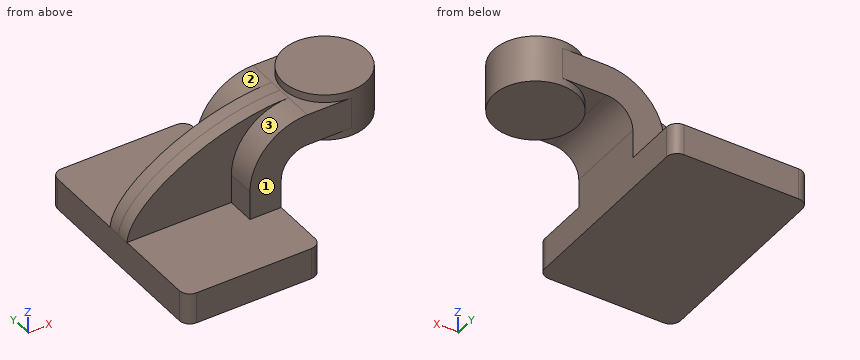
```python
from build123d import *

# Parameters (mm, degrees)
F1_DEPTH = 63.5
F0_W     = 25.4
F0_H     = 19.05
F2_DEPTH = 25.4
F3_DEPTH = 7.9375
F5_R     = 6.35


with BuildPart() as f1:
    # F0 (on Front) → F1 (new body, symmetric)
    with BuildSketch(Plane.XZ):
        Polygon((-41.275, -9.525), (41.275, -9.525), (41.275, 9.525), (22.225, 9.525), (-41.275, 9.525), align=None)
    extrude(amount=F1_DEPTH, both=True)

    # F0 (on Front) → F2 (join, symmetric)
    with BuildSketch(Plane.XZ):
        with BuildLine():
            Line((22.225, 9.525), (41.275, 9.525))
            Line((41.275, 9.525), (41.275, 27.0002))
            ThreePointArc((41.275, 27.0002), (45.9246798487, 38.2255201513), (57.15, 42.8752))
            Line((57.15, 42.8752), (58.7173181552, 42.8752))
            Line((58.7173181552, 42.8752), (58.7173181552, 61.9252))
            Line((58.7173181552, 61.9252), (57.15, 61.9252))
            ThreePointArc((57.15, 61.9252), (32.4542956671, 51.6959043329), (22.225, 27.0002))
            Line((22.225, 27.0002), (22.225, 9.525))
        make_face()
        with Locations((71.4173181552, 52.4002)):
            Rectangle(F0_W, F0_H)
    extrude(amount=F2_DEPTH, both=True)

    # F0 (on Front) → F3 (join, symmetric)
    with BuildSketch(Plane.XZ):
        with BuildLine():
            add(Edge.make_bspline(
                [(-41.275, 9.525), (-39.4876301289, 34.0806692839), (13.6961471289, 62.1632300317), (57.15, 61.9252)],
                knots=[0, 0, 0, 0, 111.5045361635, 111.5045361635, 111.5045361635, 111.5045361635], degree=3))
            Line((-41.275, 9.525), (22.225, 9.525))
            Line((22.225, 9.525), (22.225, 27.0002))
            ThreePointArc((22.225, 27.0002), (32.4542956671, 51.6959043329), (57.15, 61.9252))
        make_face()
    extrude(amount=F3_DEPTH, both=True)

    # F0 (on Front) → F4 (revolve)
    with BuildSketch(Plane.XZ):
        Polygon((84.1173181552, 66.675), (84.1173181552, 61.9252), (84.1173181552, 42.8752), (84.1173181552, 38.1), (109.5173181552, 38.1), (109.5173181552, 66.675), align=None)
    revolve(axis=Axis((84.1173181552, 0, 52.3875), (0, 0, 1)))

    # F5
    f5_edges = [f1.edges().sort_by_distance(p)[0] for p in [
        (41.275, -63.5, 0),
        (-41.275, -63.5, 0),
        (41.275, 63.5, 0),
        (-41.275, 63.5, 0),
    ]]
    fillet(f5_edges, radius=F5_R)


solid = f1.part
```
CAD build for the part. Positions are in the model's coordinates, mm. Face numbers are marked on the shaded views. A direction names the side the tool comes from. Round coordinates to 2 decimals unless told otherwise and drop trailing zeros. Write each loop counter-clockwise with the first axis right and the second up, starting at its lowest first coordinate (ties: lowest second). Pieces come first, ordered by that corner, then holes. Notation, with made-up numbers: (59, 80.25) - (90, 80.25) arc R27 cw to (90, 117.25) - close; hole circle Ø11 at (4, 39). An arc over 180 degrees is marked (long way). Write item = value, one per line. Start each with the question number.
Q1. Band-saw the part on A-A (x = 76.5). Give the cut face in (y, z) (3 decimals).
Q2. Drop flat-ended pins along their axis: pin 1 (15.5 mm diameter, centred on x = 38, z = 24, fed in from +Y); pin 2 (12 mm diameter, centred on y = -22.5, z = 33.5, fed in from -X); pin 3 (6 mm diameter, centred on x = 15.5, z = 31, fed in from -Y); pin 4 (19 mm diameter, centred on y = -13, z = 14, fed in from -X) (3 decimals). Give the stop position or say it passes through.
Q3. Which spindle directions (+Z, -Z, +X, -X, +Y, -Y) get a long thin tool onto all of the face, cutting with end or side? Do the marked faces 1, 2 and 3. Say none if no direction does.
Q4. Band-saw the part on C-C (y = -45.5). Give the cut face in (x, z) (3 decimals).
Q5. Probe L1, parallel to Y at x = 54, z = 59.5; L2, parallel to Z at x = 80, y = -3.5 (3 decimals); L3, parallel to Y at x = 14, z = 22. List the from-to ranges inside material, lowest first. Write a range as from..to.
Q6. Band-saw the part on B-B (y = -21). Give the cut face in (x, z) (3 decimals), then the cut area to 3 significant figures.
Answers below:
q1.outline = (-25.4, 42.875) - (-24.231, 42.875) - (-24.231, 38.1) - (24.231, 38.1) - (24.231, 42.875) - (25.4, 42.875) - (25.4, 61.925) - (24.231, 61.925) - (24.231, 66.675) - (-24.231, 66.675) - (-24.231, 61.925) - (-25.4, 61.925) - close
q2.pin_1 = 25.4
q2.pin_2 = 22.23
q2.pin_3 = -7.94
q2.pin_4 = -41.275
q3.face_1 = +Z, +X, -X, -Y
q3.face_2 = +Z, -X, +Y
q3.face_3 = +Z, -X, -Y
q4.outline = (-41.275, -9.525) - (41.275, -9.525) - (41.275, 9.525) - (-41.275, 9.525) - close
q5.L1 = -25.4..25.4
q5.L2 = 38.1..66.675
q5.L3 = -7.94..7.94
q6.outline = (-41.275, -9.525) - (41.275, -9.525) - (41.275, 27) arc R15.875 cw to (57.15, 42.875) - (69.829, 42.875) - (69.829, 38.1) - (98.406, 38.1) - (98.406, 66.675) - (69.829, 66.675) - (69.829, 61.925) - (57.15, 61.925) arc R34.925 ccw to (22.225, 27) - (22.225, 9.525) - (-41.275, 9.525) - close
q6.area = 3,720 mm2
